The listing builds one solid part. Answer for the finished solid, in the listing's coordinates (mm). A direction names the side the tool comes from. Round coordinates to 2 decimals unless told otherwise and drop trailing zeros. Write each loop counter-clockwise with the first axis right and the second up, starting at its lowest first coordinate (ties: lowest second). Pieces come first, ordered by that corner, then holes.
(1) For faces 1 (the face through (28.5, 20.53, -2.46)), 2 (the face through (-29.9, 9, -2)), 3 (the face through (-27.727, -2.188, -4.465)), determine the directions among +Z, -Z, +X, -X, +Y, -Y from which every point of the face is accessible in a straight line to the end or side of a thin tool.
(2) Find the intervals of material crossed by probe 1 along Y at (x, z) = (22, -5.25); probe 2 along Y at (x, z) = (-18, -3.5); probe 3 along X at (y, z) = (19, -4), in increasing order.
(3) A cutting plane is placed at B-B, the plane y = 5.5. Give the vertices of the cut face in (x, z).
(4) A cutting plane is placed at C-C, the plane z = -3.5. Give the number of separate pieces and of enclosed holes in the cut face, and give its area (3 significant figures).
(5) A cutting plane is placed at A-A, the plane x = -14.95. Give the vertices of the cut face in (y, z), and give its area (3 significant figures).
(6) Each of these flat-tipped pins is pushed along its axis until it touches: pin 1 Ø1.5 at (x, z) = (1.5, -4) entering from -Y; pin 2 Ø4 at (y, z) = (12, -2) entering from +X; pin 3 Ø1 at (x, y) = (13.5, 1) entering from +Z. Where does it stop, or does it pass through?
(7) The mould has two halves that part along X. Classify faces 4 (the face through (7.291, 18.936, -3.451)), 5 (the face through (-31.72, 23.67, -5.99)), 6 (the face through (0, 17, -7)): +X half, -X half, draft (parallel to the pull), parting line (faces both ways), or undercut.
from build123d import *

# Parameters (mm, degrees)
BOSS_EXTRUDE1_DEPTH = 5
BOSS_EXTRUDE3_DEPTH = 2
CUT_EXTRUDE1_START  = -3
CUT_EXTRUDE1_DEPTH  = 3
SKETCH4_R           = 5
SKETCH4_R_2         = 11
CUT_EXTRUDE2_DEPTH  = 44.984201709
SKETCH5_R           = 7
SKETCH5_R_2         = 5
BOSS_EXTRUDE4_DEPTH = 5
FILLET1_SIZE        = 1
FILLET1_SIZE_2      = 3


with BuildPart() as part:
    # Sketch1 → Boss-Extrude1 (new body)
    with BuildSketch(Plane.XY):
        with BuildLine():
            Line((-29.9, 17.1), (-29.9, 0.6))
            ThreePointArc((-29.9, 0.6), (-28.464823228, -2.864823228), (-25, -4.3))
            Line((-25, -4.3), (25, -4.3))
            ThreePointArc((25, -4.3), (28.464823228, -2.864823228), (29.9, 0.6))
            Line((29.9, 0.6), (29.9, 17.1))
            ThreePointArc((29.9, 17.1), (28.464823228, 20.564823228), (25, 22))
            Line((25, 22), (-25, 22))
            ThreePointArc((-25, 22), (-28.464823228, 20.564823228), (-29.9, 17.1))
        make_face()
    extrude(amount=-BOSS_EXTRUDE1_DEPTH)

    # Sketch2 → Boss-Extrude3 (add)
    with BuildSketch(Plane(origin=(0, 0, -5), x_dir=(-1, 0, 0), z_dir=(0, 0, -1))):
        with BuildLine():
            Line((34.4, 0.6), (34.4, 17.1))
            ThreePointArc((34.4, 17.1), (31.646803743, 23.746803743), (25, 26.5))
            Line((25, 26.5), (-25, 26.5))
            ThreePointArc((-25, 26.5), (-31.646803743, 23.746803743), (-34.4, 17.1))
            Line((-34.4, 17.1), (-34.4, 0.6))
            ThreePointArc((-34.4, 0.6), (-31.646803743, -6.046803743), (-25, -8.8))
            Line((-25, -8.8), (25, -8.8))
            ThreePointArc((25, -8.8), (31.646803743, -6.046803743), (34.4, 0.6))
        make_face()
        with BuildLine():
            Line((28.9, 0.6), (28.9, 17.1))
            ThreePointArc((28.9, 17.1), (27.757716447, 19.857716447), (25, 21))
            Line((25, 21), (-25, 21))
            ThreePointArc((-25, 21), (-27.757716447, 19.857716447), (-28.9, 17.1))
            Line((-28.9, 17.1), (-28.9, 0.6))
            ThreePointArc((-28.9, 0.6), (-27.757716447, -2.157716447), (-25, -3.3))
            Line((-25, -3.3), (25, -3.3))
            ThreePointArc((25, -3.3), (27.757716447, -2.157716447), (28.9, 0.6))
        make_face(mode=Mode.SUBTRACT)
    extrude(amount=BOSS_EXTRUDE3_DEPTH)

    # Sketch3 → Cut-Extrude1 (cut)
    with BuildSketch(Plane(origin=(0, 0, -5), x_dir=(-1, 0, 0), z_dir=(0, 0, -1)).offset(CUT_EXTRUDE1_START)):
        with BuildLine():
            Line((-25, -3.3), (25, -3.3))
            ThreePointArc((25, -3.3), (27.757716447, -2.157716447), (28.9, 0.6))
            Line((28.9, 0.6), (28.9, 17.1))
            ThreePointArc((28.9, 17.1), (27.757716447, 19.857716447), (25, 21))
            Line((25, 21), (-25, 21))
            ThreePointArc((-25, 21), (-27.757716447, 19.857716447), (-28.9, 17.1))
            Line((-28.9, 17.1), (-28.9, 0.6))
            ThreePointArc((-28.9, 0.6), (-27.757716447, -2.157716447), (-25, -3.3))
        make_face()
    extrude(amount=CUT_EXTRUDE1_DEPTH, mode=Mode.SUBTRACT)

    # Sketch4 → Cut-Extrude2 (cut, through all)
    with BuildSketch(Plane.XY):
        with Locations((4.983333333, 14.5)):
            Circle(SKETCH4_R)
        with Locations((-14.95, 8.85)):
            Circle(SKETCH4_R_2)
        with Locations((19.933333333, 12)):
            Circle(SKETCH4_R)
    extrude(amount=-CUT_EXTRUDE2_DEPTH, mode=Mode.SUBTRACT)

    # Sketch5 → Boss-Extrude4 (add)
    with BuildSketch(Plane(origin=(0, 0, -2), x_dir=(-1, 0, 0), z_dir=(0, 0, -1))):
        with Locations((-4.983333333, 14.5)):
            Circle(SKETCH5_R)
        with Locations(Location((-4.983333333, 14.5, 0), (0, 0, 180))):
            Circle(SKETCH5_R_2, mode=Mode.SUBTRACT)
    extrude(amount=BOSS_EXTRUDE4_DEPTH)

    # Fillet1
    # an asymmetric fillet: 3, 1 mm, written as the material it adds along each edge
    with BuildSketch(Plane(origin=(4.983333333, 14.5, -2), x_dir=(-0.6399684103972102, 0.7684012192166719, 0), z_dir=(-0.7684012192166719, -0.6399684103972102, 0))) as fillet1_piece_1_section:
        with BuildLine():
            Bezier((7 + FILLET1_SIZE, 0), (7, 0), (7, FILLET1_SIZE_2), weights=[1, 0.707106781, 1])
            Line((7, FILLET1_SIZE_2), (7, 0))
            Line((7, 0), (7 + FILLET1_SIZE, 0))
        make_face()
    fillet1_piece_1 = revolve(axis=Axis((4.983333333, 14.5, -2), (0, 0, -1)), revolution_arc=309.789463983, mode=Mode.PRIVATE)
    fillet1_piece_1 = split(fillet1_piece_1, bisect_by=Plane(origin=(1.135555839, 21, -2.732538618), z_dir=(0, -1, 0)), keep=Keep.TOP, mode=Mode.PRIVATE)
    add(fillet1_piece_1)
    with BuildSketch(Plane(origin=(4.983333333, 14.5, -2), x_dir=(-1, 0, 0), z_dir=(0, -1, 0))) as fillet1_piece_2_section:
        with BuildLine():
            Bezier((7 + FILLET1_SIZE, 0), (7, 0), (7, FILLET1_SIZE_2), weights=[1, 0.707106781, 1])
            Line((7, FILLET1_SIZE_2), (7, 0))
            Line((7, 0), (7 + FILLET1_SIZE, 0))
        make_face()
    fillet1_piece_2 = revolve(axis=Axis((4.983333333, 14.5, -2), (0, 0, -1)), revolution_arc=129.61571024, mode=Mode.PRIVATE)
    fillet1_piece_2 = split(fillet1_piece_2, bisect_by=Plane(origin=(-1.041526042, 21, -2.873194596), z_dir=(0, -1, 0)), keep=Keep.TOP, mode=Mode.PRIVATE)
    add(fillet1_piece_2)


solid = part.part
Solutions:
1. face 1: +Z, +X, +Y
1. face 2: +Z, -X, +Y, -Y
1. face 3: -Z
2. probe 1: y = -8.8 to -3.3, 21 to 26.5
2. probe 2: y = -4.3 to -3.3, 21 to 22
2. probe 3: x = -29.52 to -28.41, -0.45 to 2.8, 7.16 to 10.42, 28.41 to 29.52
3. outline: (-34.4, -7) - (-28.9, -7) - (-28.9, -2) - (-25.43, -2) - (-25.43, 0) - (-29.9, 0) - (-29.9, -5) - (-34.4, -5) - close; (-4.47, -2) - (28.9, -2) - (28.9, -7) - (34.4, -7) - (34.4, -5) - (29.9, -5) - (29.9, 0) - (-4.47, 0) - close
4. separate pieces: 1
4. enclosed holes: 2
4. area: 239 mm2
5. outline: (-8.8, -7) - (-3.3, -7) - (-3.3, -2) - (-2.15, -2) - (-2.15, 0) - (-4.3, 0) - (-4.3, -5) - (-8.8, -5) - close; (19.85, -2) - (21, -2) - (21, -7) - (26.5, -7) - (26.5, -5) - (22, -5) - (22, 0) - (19.85, 0) - close
5. area: 36.6 mm2
6. pin 1: stops at y = -4.3
6. pin 2: stops at x = 29.9
6. pin 3: stops at z = 0
7. face 4: undercut
7. face 5: -X half
7. face 6: draft
